from build123d import *

# Parameters (mm, degrees)
SZKIC1_W                    = 4.78
SZKIC1_H                    = 4.78
DODANIE_WYCI_GNI_CIE1_DEPTH = 36
ZAOKR_GLENIE1_RADIUS        = 2.39
ZAOKR_GLENIE1_LENGTH        = 4.78
ZAOKR_GLENIE2_RADIUS        = 2.39
ZAOKR_GLENIE2_LENGTH        = 4.78


with BuildPart() as part:
    # Szkic1 → Dodanie-wyciągnięcie1 (new body)
    with BuildSketch(Plane.XY):
        Rectangle(SZKIC1_W, SZKIC1_H)
    extrude(amount=DODANIE_WYCI_GNI_CIE1_DEPTH)

    # Zaokrąglenie1: full round fillet: the end face becomes a half cylinder, R = half its width
    zaokr_glenie1_face = Plane((0, 0, 36), x_dir=(-1, 0, 0), z_dir=(0, 0, 1))  # on the end face: x along it, z out of the body
    zaokr_glenie1_slab = zaokr_glenie1_face.offset(-ZAOKR_GLENIE1_RADIUS / 2) * Box(ZAOKR_GLENIE1_LENGTH, 2 * ZAOKR_GLENIE1_RADIUS, ZAOKR_GLENIE1_RADIUS, mode=Mode.PRIVATE)  # the body's end, R deep
    zaokr_glenie1_round = Plane((0, 0, 33.61), x_dir=(0, 0, 1), z_dir=(-1, 0, 0)) * Cylinder(ZAOKR_GLENIE1_RADIUS, ZAOKR_GLENIE1_LENGTH, mode=Mode.PRIVATE)  # its axis R under the face
    add(zaokr_glenie1_slab - zaokr_glenie1_round, mode=Mode.SUBTRACT)

    # Zaokrąglenie2: full round fillet: the end face becomes a half cylinder, R = half its width
    zaokr_glenie2_face = Plane((0, 0, 0), x_dir=(1, 0, 0), z_dir=(0, 0, -1))  # on the end face: x along it, z out of the body
    zaokr_glenie2_slab = zaokr_glenie2_face.offset(-ZAOKR_GLENIE2_RADIUS / 2) * Box(ZAOKR_GLENIE2_LENGTH, 2 * ZAOKR_GLENIE2_RADIUS, ZAOKR_GLENIE2_RADIUS, mode=Mode.PRIVATE)  # the body's end, R deep
    zaokr_glenie2_round = Plane((0, 0, 2.39), x_dir=(0, 0, -1), z_dir=(1, 0, 0)) * Cylinder(ZAOKR_GLENIE2_RADIUS, ZAOKR_GLENIE2_LENGTH, mode=Mode.PRIVATE)  # its axis R under the face
    add(zaokr_glenie2_slab - zaokr_glenie2_round, mode=Mode.SUBTRACT)


solid = part.part
Design review of the part built by this model. Coordinates are the model's own, in mm. Round coordinates to 2 decimals unless told otherwise and drop trailing zeros. Write each loop counter-clockwise with the first axis right and the second up, starting at its lowest first coordinate (ties: lowest second). Pieces come first, ordered by that corner, then holes. Notation, with made-up numbers: (14.25, -39) -> (68.25, -39) arc R7 cw to (68.25, -27) -> close; hole circle Ø3 at (-12, 0). An arc over 180 degrees is marked (long way). One line per question, with ' | ' between items.
(1) Insertion check: P1, Ø2, axis at x = 1.5, y = -1.5, coming from the +Z side. The pin has a flat end and moves straight along its axis. Give the tip position at first contact, or say it passes through.
Result sheet:
P1: z = 35.95
(2) Wall thickness on line 1 (Z direction, x = -1.7, y = -1.45); line 2 (Y direction, x = -1.4, z = 34.5); line 3 (Z direction, x = 0.9, y = -1): over which ranges is each line inside the solid? List them lowest first. Write a range as [from, to].
Result sheet:
line 1: [0.49, 35.51] | line 2: [-2.22, 2.22] | line 3: [0.22, 35.78]
(3) Take a section at B-B, the plane y = 1.7. State the section outline as (x, z) points.
Result sheet:
outline: (-2.39, 0.71) -> (2.39, 0.71) -> (2.39, 35.29) -> (-2.39, 35.29) -> close
(4) Take a section at A-A, the plane x = -0.6. State the section outline as (y, z) points.
Result sheet:
outline: (-2.39, 2.39) arc R2.39 ccw to (2.39, 2.39) -> (2.39, 33.61) arc R2.39 ccw to (-2.39, 33.61) -> close
